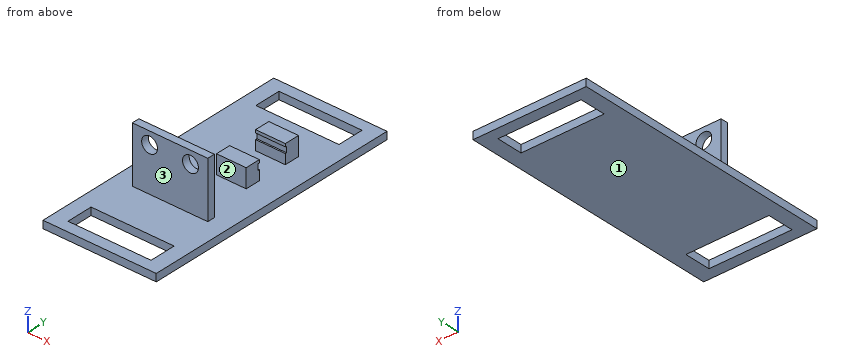
```python
from build123d import *

# Parameters (mm, degrees)
F1_W      = 38.1
F1_H      = 88.9
F2_DEPTH  = 2.54
F0_W      = 10
F0_H      = 5.08
F0_W_2    = 25.4
F0_H_2    = 2.54
F3_DEPTH  = 6.35
F4_W      = 10
F4_H      = 2
F5_DEPTH  = 0.5
F6_W      = 10
F6_H      = 2
F7_DEPTH  = 0.5
F8_DEPTH  = 12.7
F9_R      = 2.665
F10_DEPTH = 61.9361865292
F11_W     = 27.94
F11_H     = 8.89
F12_DEPTH = 25.4


with BuildPart() as f2:
    # F1 (on Top) → F2 (new body)
    with BuildSketch(Plane.XY):
        with Locations((19.05, 44.45)):
            Rectangle(F1_W, F1_H)
    extrude(amount=-F2_DEPTH)

    # F0 (on Top) → F3 (join)
    with BuildSketch(Plane.XY):
        with Locations((24.05, 62.6320488313)):
            Rectangle(F0_W, F0_H)
        with Locations((24.05, 47.5520488313)):
            Rectangle(F0_W, F0_H)
        with Locations((19.1884456806, 28.2348134708)):
            Rectangle(F0_W_2, F0_H_2)
    extrude(amount=F3_DEPTH)

    # F4 (on face) → F5 (cut)
    with BuildSketch(Plane(origin=(0, 50.0920488313, 0), x_dir=(-1, 0, 0), z_dir=(0, 1, 0))):
        with Locations((-24.05, 4.35)):
            Rectangle(F4_W, F4_H)
    extrude(amount=-F5_DEPTH, mode=Mode.SUBTRACT)

    # F6 (on face) → F7 (cut)
    with BuildSketch(Plane.XZ.offset(-60.0920488313)):
        with Locations((24.05, 4.35)):
            Rectangle(F6_W, F6_H)
    extrude(amount=-F7_DEPTH, mode=Mode.SUBTRACT)

    # F8 (add): a face of the model
    f8_faces = [f2.faces().sort_by_distance(p)[0] for p in [
        (19.1884456806, 28.2348134708, 6.35),
    ]]
    extrude(f8_faces, amount=F8_DEPTH)

    # F9 (on face) → F10 (cut, through all)
    with BuildSketch(Plane.XZ.offset(-26.9648134708)):
        with Locations((12.3068671674, 14.8589983582)):
            Circle(F9_R)
        with Locations((26.0700241938, 14.8589983582)):
            Circle(F9_R)
    extrude(amount=-F10_DEPTH, mode=Mode.SUBTRACT)

    # F11 (on face) → F12 (cut)
    with BuildSketch(Plane.XY):
        with Locations((19.05, 80.645)):
            Rectangle(F11_W, F11_H)
        with Locations((19.05, 8.255)):
            Rectangle(F11_W, F11_H)
    extrude(amount=-F12_DEPTH, mode=Mode.SUBTRACT)


solid = f2.part
```
Read the model definition and answer for the solid it produces. Units are mm, in the model's axes. Face numbers are marked on the shaded views. Coordinates: 2 decimals unless noted, no trailing zeros. Order: outer loops, then holes, each group sorted by start corner. A loop starts at its lowest first (then second) coordinate and runs counter-clockwise, first axis right, second up. Notation, with made-up numbers: (72.5, -19) - (99.5, -19) arc R22 cw to (99.5, -10) - close; hole circle Ø3 at (80.5, 36). An arc over 180 degrees is marked (long way). Answer as a JSON object with one key per item and string values. Group by question number.
Item 1: Consider probe 1 along Y at (x, z) = (23, 5.25); probe 2 along Y at (x, z) = (23, -1); probe 3 along Y at (x, z) = (16, 14.5). Determine where each line is inside the solid, lowest interval first. Write a range as from..to.
Item 2: Section A-A (x = 30.5) is taken. Give the vertices of the cut face in (y, z), plus the area to 3 significant figures.
Item 3: Section D-D (x = 11) is taken. Give the vertices of the cut face in (y, z), plus the area to 3 significant figures.
Item 4: The mould has two halves that part along Y. Classify the marked faces 1, 2 and 3: +Y half, -Y half, draft (parallel to the pull), parting line (faces both ways), or undercut.
Item 5: Section C-C (z = 16) is taken. Give the vertices of the cut face in (x, y).
Item 6: Section B-B (y = 81) is taken. Give the vertices of the cut face in (x, z), plus the area to 3 significant figures.
Item 7: Flat-ended cylindrical pins translate along their axes: P1, Ø5, axis at x = 5.5, z = 9.5, coming from the -Y side; P2, Ø2.5, axis at y = 48, z = 2.5, coming from the -X side; P3, Ø2.5, axis at x = 25, y = 47, coming from the +Z side; P4, Ø2, axis at y = 10.5, z = -1.5, coming from the -X side. Find the tip coordinate at first contact, or state that the pin passes through.
Results are:
{
 "1": {"probe 1": "y = 26.96..29.5, 45.01..49.59, 60.59..65.17", "probe 2": "y = 0..3.81, 12.7..76.2, 85.09..88.9", "probe 3": "y = 26.96..29.5"},
 "2": {"outline": "(0, -2.54) - (3.81, -2.54) - (3.81, 0) - (0, 0) - close; (12.7, -2.54) - (76.2, -2.54) - (76.2, 0) - (29.5, 0) - (29.5, 19.05) - (26.96, 19.05) - (26.96, 0) - (12.7, 0) - close; (85.09, -2.54) - (88.9, -2.54) - (88.9, 0) - (85.09, 0) - close", "area": "229 mm^2"},
 "3": {"outline": "(0, -2.54) - (3.81, -2.54) - (3.81, 0) - (0, 0) - close; (12.7, -2.54) - (76.2, -2.54) - (76.2, 0) - (29.5, 0) - (29.5, 12.54) - (26.96, 12.54) - (26.96, 0) - (12.7, 0) - close; (26.96, 17.18) - (29.5, 17.18) - (29.5, 19.05) - (26.96, 19.05) - close; (85.09, -2.54) - (88.9, -2.54) - (88.9, 0) - (85.09, 0) - close", "area": "217 mm^2"},
 "4": {"face 1": "draft", "face 2": "undercut", "face 3": "-Y half"},
 "5": {"outline": "(6.49, 26.96) - (9.9, 26.96) - (9.9, 29.5) - (6.49, 29.5) - close; (14.72, 26.96) - (23.66, 26.96) - (23.66, 29.5) - (14.72, 29.5) - close; (28.48, 26.96) - (31.89, 26.96) - (31.89, 29.5) - (28.48, 29.5) - close"},
 "6": {"outline": "(0, -2.54) - (5.08, -2.54) - (5.08, 0) - (0, 0) - close; (33.02, -2.54) - (38.1, -2.54) - (38.1, 0) - (33.02, 0) - close", "area": "25.8 mm^2"},
 "7": {"P1": "stops at y = 26.96", "P2": "stops at x = 19.05", "P3": "stops at z = 6.35", "P4": "stops at x = 0"}
}
